```python
from build123d import *

# Parameters (mm, degrees)
SKETCH1_W                    = 130
SKETCH1_H                    = 1700
BASE_FLANGE1_DEPTH           = 2
EDGE_FLANGE1_STRIP_W         = 13
EDGE_FLANGE1_STRIP_H         = 2
EDGE_FLANGE1_STRIP_CUT_DEPTH = 1700
EDGE_FLANGE1_DEPTH           = 1700
EDGE_FLANGE2_STRIP_W         = 13
EDGE_FLANGE2_STRIP_H         = 2
EDGE_FLANGE2_STRIP_CUT_DEPTH = 1700
EDGE_FLANGE2_DEPTH           = 1700
EDGE_FLANGE3_STRIP_W         = 12
EDGE_FLANGE3_STRIP_H         = 2
EDGE_FLANGE3_STRIP_CUT_DEPTH = 1700
EDGE_FLANGE3_DEPTH           = 1700
CUT_EXTRUDE1_DEPTH           = 1415.486194049
CUT_EXTRUDE1_DEPTH_BACK      = 1415.486194049
SKETCH15_W                   = 28
SKETCH15_H                   = 30
SKETCH16_R                   = 4
CUT_EXTRUDE2_DEPTH           = 10


# Sheet-metal steps are written as plain solids
with BuildPart() as part:
    # Sketch1 → Base-Flange1 (new body)
    with BuildSketch(Plane.XY):
        with Locations((36.609195402, -556.379310345)):
            Rectangle(SKETCH1_W, SKETCH1_H)
    extrude(amount=-BASE_FLANGE1_DEPTH)

    # Edge-Flange1 strip (across the edge) → Edge-Flange1 strip cut (cut)
    with BuildSketch(Plane(origin=(101.609195402, -1406.379310345, 0), x_dir=(-1, 0, 0), z_dir=(0, 1, 0))):
        with Locations((-2, -1)):
            Rectangle(EDGE_FLANGE1_STRIP_W, EDGE_FLANGE1_STRIP_H)
    extrude(amount=EDGE_FLANGE1_STRIP_CUT_DEPTH, mode=Mode.SUBTRACT)

    # Edge-Flange1 section (across the edge) → Edge-Flange1 (add)
    with BuildSketch(Plane(origin=(101.609195402, -1406.379310345, 0), x_dir=(-1, 0, 0), z_dir=(0, 1, 0))):
        with BuildLine():
            Line((0, 2.5), (0, 13))
            Line((0, 13), (2, 13))
            Line((2, 13), (2, 2.5))
            ThreePointArc((2, 2.5), (2.732233047, 0.732233047), (4.5, 0))
            Line((4.5, 0), (4.5, -2))
            ThreePointArc((4.5, -2), (1.318019485, -0.681980515), (0, 2.5))
        make_face()
    extrude(amount=EDGE_FLANGE1_DEPTH)

    # Edge-Flange2 strip (across the edge) → Edge-Flange2 strip cut (cut)
    with BuildSketch(Plane(origin=(-28.390804598, 293.620689655, 0), x_dir=(1, 0, 0), z_dir=(0, -1, 0))):
        with Locations((-2, -1)):
            Rectangle(EDGE_FLANGE2_STRIP_W, EDGE_FLANGE2_STRIP_H)
    extrude(amount=EDGE_FLANGE2_STRIP_CUT_DEPTH, mode=Mode.SUBTRACT)

    # Edge-Flange2 section (across the edge) → Edge-Flange2 (add)
    with BuildSketch(Plane(origin=(-28.390804598, 293.620689655, 0), x_dir=(1, 0, 0), z_dir=(0, -1, 0))):
        with BuildLine():
            Line((0, 2.5), (0, 108))
            Line((0, 108), (2, 108))
            Line((2, 108), (2, 2.5))
            ThreePointArc((2, 2.5), (2.732233047, 0.732233047), (4.5, 0))
            Line((4.5, 0), (4.5, -2))
            ThreePointArc((4.5, -2), (1.318019485, -0.681980515), (0, 2.5))
        make_face()
    extrude(amount=EDGE_FLANGE2_DEPTH)

    # Edge-Flange3 strip (across the edge) → Edge-Flange3 strip cut (cut)
    with BuildSketch(Plane(origin=(-28.390804598, -1406.379310345, 108), x_dir=(0, 0, -1), z_dir=(0, 1, 0))):
        with Locations((-4, -1)):
            Rectangle(EDGE_FLANGE3_STRIP_W, EDGE_FLANGE3_STRIP_H)
    extrude(amount=EDGE_FLANGE3_STRIP_CUT_DEPTH, mode=Mode.SUBTRACT)

    # Edge-Flange3 section (across the edge) → Edge-Flange3 (add)
    with BuildSketch(Plane(origin=(-28.390804598, -1406.379310345, 108), x_dir=(0, 0, -1), z_dir=(0, 1, 0))):
        with BuildLine():
            Line((-2, 2), (-2, 30))
            Line((-2, 30), (0, 30))
            Line((0, 30), (0, 2))
            ThreePointArc((0, 2), (0.585786438, 0.585786438), (2, 0))
            Line((2, 0), (2, -2))
            ThreePointArc((2, -2), (-0.828427125, -0.828427125), (-2, 2))
        make_face()
    extrude(amount=EDGE_FLANGE3_DEPTH)

    # Sketch15 → Cut-Extrude1 (cut, two sides: drawn at the far end of the back side and taken through both)
    with BuildSketch(Plane.XY.offset(110).offset(-CUT_EXTRUDE1_DEPTH_BACK)):
        with Locations((-44.390804598, -1391.379310345)):
            Rectangle(SKETCH15_W, SKETCH15_H)
        with Locations((-44.390804598, 278.620689655)):
            Rectangle(SKETCH15_W, SKETCH15_H)
    extrude(amount=CUT_EXTRUDE1_DEPTH + CUT_EXTRUDE1_DEPTH_BACK, mode=Mode.SUBTRACT)

    # Sketch16 → Cut-Extrude2 (cut)
    with BuildSketch(Plane.XY.offset(110)):
        with Locations((-42.390804598, -1226.379310345)):
            Circle(SKETCH16_R)
        with Locations((-42.390841166, -556.379310345)):
            Circle(SKETCH16_R)
        with Locations((-42.390877735, 113.620689655)):
            Circle(SKETCH16_R)
    extrude(amount=-CUT_EXTRUDE2_DEPTH, mode=Mode.SUBTRACT)


solid = part.part
```
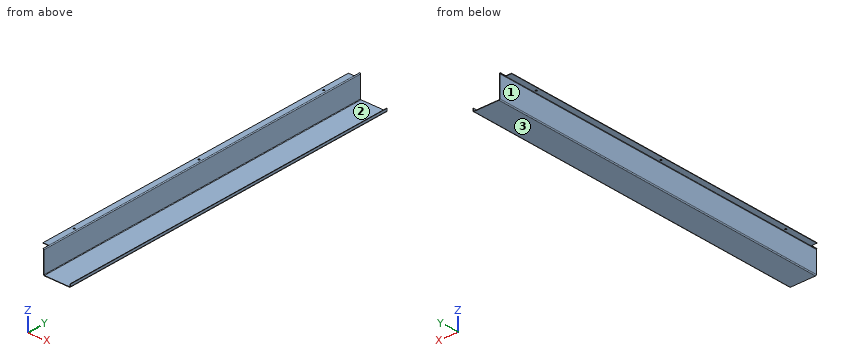
Source: CAD feature listing. Evaluate the final solid. Frame: model axes, mm. Face numbers are marked on the shaded views. Coordinates: 2 decimals unless noted, no trailing zeros. Loops run counter-clockwise (first coordinate to the right, second up) from the corner with the lowest first, then second, coordinate; pieces in that order, holes last. Notation, with made-up numbers: (-11.5, 20) -> (9.5, 20) arc R16 cw to (9.5, 28) -> close; hole circle Ø4 at (-35, -15). An arc over 180 degrees is marked (long way). One line per item, written item: value. Start each with the question number.
Q1. Contact query for flat-ended pins moving along their axis: P1, Ø1.5, axis at y = -110.5, z = 36, coming from the +X side; P2, Ø6, axis at y = -88, z = 14.5, coming from the -X side; P3, Ø2, axis at x = -40.5, z = 109.5, coming from the -Y side. Output: stop coordinate, or through.
Q2. Mould query, pull axis X, two halves, no side actions, for the marked faces 1, 2 and 3. Classes: pulls with the +X half, pulls with the -X half, needs draft (parallel to the pull), parting line crosses it, or undercut.
Q3. Section query A-A, the plane y = -1110. Return the cut outline in (x, z).
Q4. Section query B-B, the plane z = 41. Return the cut outline in (x, y), and give its area (3 significant figures).
Q5. Line query: line 1 along Z through (x, y) = (-30.5, -708.5); line 2 along Z through (x, y) = (70, -1281.5); line 3 along X through (y, z) = (-484, 37). Output: solid intervals per line, ascending.
Q6. Section query C-C, the plane x = 29.5. Return the cut outline in (y, z).
Results:
1. P1: x = -26.39
1. P2: x = -28.39
1. P3: y = -1376.38
2. face 1: pulls with the -X half
2. face 2: undercut
2. face 3: needs draft
3. outline: (-58.39, 108) -> (-30.39, 108) arc R2 cw to (-28.39, 106) -> (-28.39, 2.5) arc R4.5 ccw to (-23.89, -2) -> (97.11, -2) arc R4.5 ccw to (101.61, 2.5) -> (101.61, 13) -> (99.61, 13) -> (99.61, 2.5) arc R2.5 cw to (97.11, 0) -> (-23.89, 0) arc R2.5 cw to (-26.39, 2.5) -> (-26.39, 106) arc R4 ccw to (-30.39, 110) -> (-58.39, 110) -> close
4. outline: (-28.39, -1406.38) -> (-26.39, -1406.38) -> (-26.39, 293.62) -> (-28.39, 293.62) -> close
4. area: 3,400 mm^2
5. line 1: 108 to 110
5. line 2: -2 to 0
5. line 3: -28.39 to -26.39
6. outline: (-1406.38, -2) -> (293.62, -2) -> (293.62, 0) -> (-1406.38, 0) -> close
